Design review of the part built by this model. Coordinates are the model's own, in mm. A direction names the side the tool comes from. Give positions to 0.01 mm unless a question says otherwise; leave off trailing zeros. Write each loop counter-clockwise with the first axis right and the second up, starting at its lowest first coordinate (ties: lowest second). Pieces come first, ordered by that corner, then holes. Notation, with made-up numbers: M 67,6 L 111,6 A29 ccw 111,35 Z; hole C 53.5,-2.5 d9. An arc over 180 degrees is marked long. One line per item, written item: value. Start each with the question number.
```python
from build123d import *

# Parameters (mm, degrees)
F1_DEPTH = 25
F2_T     = -2
F4_DEPTH = 20.3


with BuildPart() as f1:
    # F0 (on Top) → F1 (new body)
    with BuildSketch(Plane.XY):
        with BuildLine():
            Line((64.2109500094, 12.4102973465), (2.3917296289, 19.8564757543))
            ThreePointArc((2.3917296289, 19.8564757543), (-20, 0), (2.3917296289, -19.8564757543))
            Line((2.3917296289, -19.8564757543), (64.2109500094, -12.4102973465))
            ThreePointArc((64.2109500094, -12.4102973465), (75.2161189914, 0), (64.2109500094, 12.4102973465))
        make_face()
    extrude(amount=F1_DEPTH)

    # F2
    f2_openings = [f1.faces().sort_by_distance(p)[0] for p in [
        (24.189424, 0, 25),
    ]]
    offset(amount=F2_T, openings=f2_openings)

    # F3 (on Front) → F4 (cut, symmetric)
    with BuildSketch(Plane.XZ):
        with BuildLine():
            ThreePointArc((59.8595843924, 9.6312405885), (34.5198825437, 20.8955157603), (6.9537251321, 23.9107024015))
            ThreePointArc((6.9537251321, 23.9107024015), (3.5680113506, 20.244996686), (7.1925410007, 16.8152385285))
            ThreePointArc((7.1925410007, 16.8152385285), (32.5850479445, 13.7268921567), (56.0830972065, 3.6195199423))
            ThreePointArc((56.0830972065, 3.6195199423), (60.9410990793, 4.7598155213), (59.8595843924, 9.6312405885))
        make_face()
    extrude(amount=F4_DEPTH, both=True, mode=Mode.SUBTRACT)


solid = f1.part
```
Q1. Wall thickness on line 1 (Y direction, x = 0, z = 20); line 2 (X direction, y = 0, z = 9.5); line 3 (Z direction, x = 65.5, y = 3): over which ranges is each line inside the solid? List them lowest first. Write a range as from..to.
Q2. Take a section at A-A, the plane x = 23. Give the boundary of the cut face in (y, z), then the cut area to 3 significant figures.
Q3. Take a section at D-D, the plane x = 0. Give the boundary of the cut face in (y, z), then the cut area to 3 significant figures.
Q4. For P1, Ø1.5, axis at x = 63.5, y = 12.5, coming from the -Z side; P2, Ø6, axis at x = 10.5, y = 5, coming from the +Z side; P3, Ø1, axis at y = 9.5, z = 9.5, coming from the -X side; P4, Ø1.5, axis at x = 11.5, z = 14, coming from the +Y side, all flat-tipped, find the tip position at first contact; note any pin that passes through.
Q5. Take a section at B-B, the plane z = 8. Give the boundary of the cut face in (x, y), then the cut area to 3 significant figures.
Q6. Take a section at C-C, the plane y = 0. Give the boundary of the cut face in (x, z), then the cut area to 3 significant figures.
Q7. The part is to be moulded in two halves that separate along Y. For faces 1 (the face through (34.65, -14.82, 20.86)), 2 (the face through (27, 0, 2)), 3 (the face through (75.214, -0.254, 12.325)), say which applies: pulls with the +Y half, pulls with the -Y half, needs draft (parallel to the pull), parting line crosses it, or undercut.
Q8. Machinability: for faces 4 (the face through (33.73, 16.08, 9.55)), 5 (the face through (34.65, 15.09, 20.86)), 6 (the face through (33.495, 14.096, 10.783)), which of the approach directions +Z, -Z, +X, -X, +Y, -Y give a long, thin tool a straight path to every point of the face, cutting with its end or side? Answer none if there is none.
Results list:
1. line 1: y = -20..-18, 18..20
1. line 2: x = -20..-18, 73.22..75.22
1. line 3: z = 0..2
2. outline: M -17.37,0 L 17.37,0 L 17.37,15.76 L 15.36,15.76 L 15.36,2 L -15.36,2 L -15.36,15.76 L -17.37,15.76 Z; M -17.37,23.21 L -15.36,23.21 L -15.36,25 L -17.37,25 Z; M 15.36,23.21 L 17.37,23.21 L 17.37,25 L 15.36,25 Z
2. area: 132 mm^2
3. outline: M -20,0 L 20,0 L 20,25 L 18,25 L 18,2 L -18,2 L -18,25 L -20,25 Z
3. area: 172 mm^2
4. P1: stops at z = 0
4. P2: stops at z = 2
4. P3: stops at x = -17.86
4. P4: stops at y = 18.85
5. outline: M 2.15,-17.87 A18 cw long 2.15,17.87 L 48.02,12.35 L 48.02,14.36 L 2.39,19.86 A20 ccw long 2.39,-19.86 L 48.02,-14.36 L 48.02,-12.35 Z; M 61.22,-12.77 L 64.21,-12.41 A12.5 ccw 64.21,12.41 L 61.22,12.77 L 61.22,10.76 L 63.97,10.42 A10.5 cw 63.97,-10.42 L 61.22,-10.76 Z
5. area: 391 mm^2
6. outline: M -20,0 L 75.22,0 L 75.22,25 L 73.22,25 L 73.22,2 L -18,2 L -18,25 L -20,25 Z
6. area: 282 mm^2
7. face 1: needs draft
7. face 2: undercut
7. face 3: parting line crosses it
8. face 4: +Z, -Z, +X, +Y
8. face 5: +Y, -Y
8. face 6: +Z
